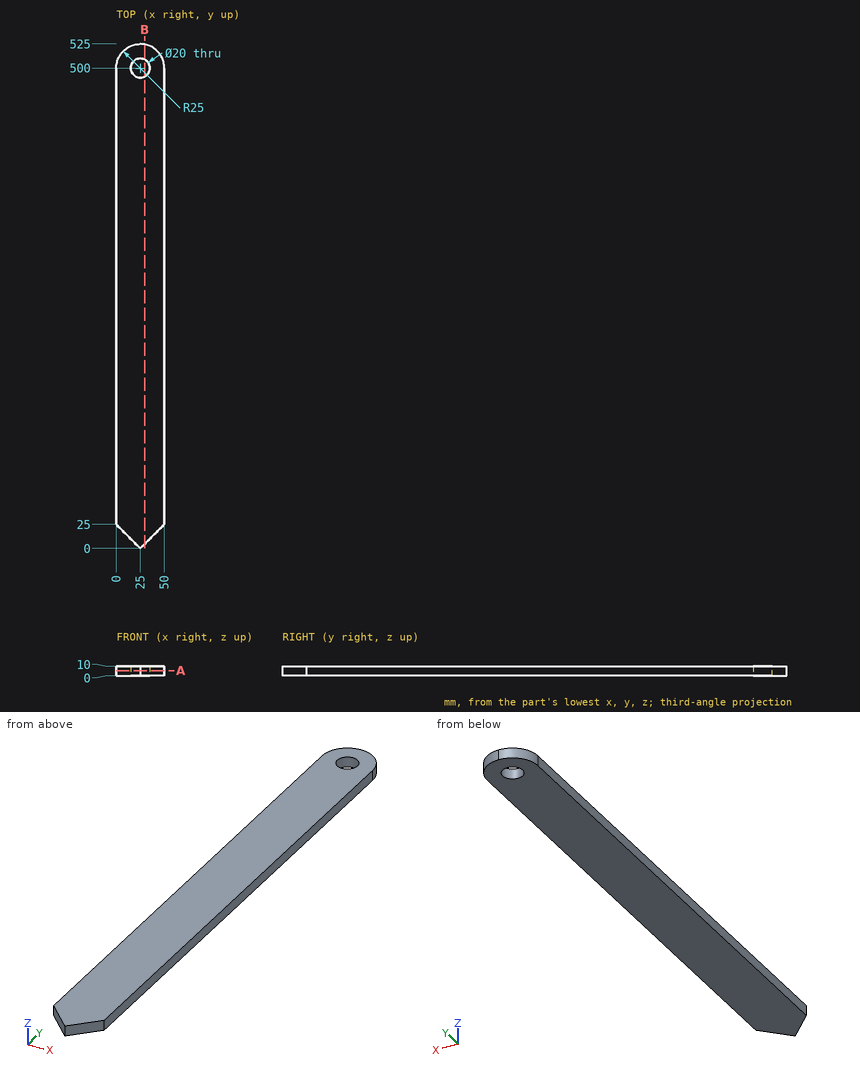
Design review of the part shown in the three views and the two pictorial views. Dimensions are in mm from the part's minimum x, y and z. Give positions to 0.01 mm unless a question says otherwise; leave off trailing zeros. Order: outer loops, then holes, each group sorted by start corner. A loop starts at its lowest first (then second) coordinate and runs counter-clockwise, first axis right, second up. Notation, with made-up numbers: M 33.5,45.25 L 62.5,45.25 A20 cw 62.5,80.25 Z; hole C -5,-5 d6. An arc over 180 degrees is marked long. Answer in a Markdown table with one row per item. Add a question column.
(1) Consider section A-A on z = 5.5. State the section outline as (x, y) points.
(2) Consider section B-B on x = 29.5. State the section outline as (y, z) points.
(3) For pin 1 (5 mm diameter, centred on x = 38.5, z = 5.5, fed in from +Y); pin 2 (1.5 mm diameter, centred on x = 44.5, z = 5, fed in from +Y); pin 3 (6 mm diameter, centred on x = 21.5, z = 3, fed in from +Y) (3 decimals), all flat-tipped, find the tip position at first contact; note any pin that passes through.
(4) Wall thickness on probe 1 along X at (y, z) = (500, 3.5); probe 2 along Y at (x, z) = (30.5, 4.25); probe 3 along Y at (x, z) = (22.5, 0.75): over which ranges is each line inside the solid? List them lowest first. Write a range as [from, to].
Evaluation:
| question | item | result |
|---|---|---|
| 1 | outline | M 0,25 L 25,0 L 50,25 L 50,500 A25 ccw 0,500 Z; hole C 25,500 d20 |
| 2 | outline | M 4.5,0 L 491.07,0 L 491.07,10 L 4.5,10 Z; M 508.93,0 L 524.59,0 L 524.59,10 L 508.93,10 Z |
| 3 | pin 1 | stops at y = 522.45 |
| 3 | pin 2 | stops at y = 516.54 |
| 3 | pin 3 | stops at y = 524.995 |
| 4 | probe 1 | x = [0, 15], [35, 50] |
| 4 | probe 2 | y = [5.5, 491.65], [508.35, 524.39] |
| 4 | probe 3 | y = [2.5, 490.32], [509.68, 524.87] |
